CAD build for the part. Positions are in the model's coordinates, mm. Face numbers are marked on the shaded views. A direction names the side the tool comes from. Coordinates: 2 decimals unless noted, no trailing zeros. Loops run counter-clockwise (first coordinate to the right, second up) from the corner with the lowest first, then second, coordinate; pieces in that order, holes last.
1) Saw through at D-D, the plane z = -170. Give the number of separate pieces and of enclosed holes in the cut face, and give its area (3 significant figures).
2) Pin check, flat tips, straight feed: pin 1 Ø4 at (x, y) = (111.5, 10.5) entering from -Z; pin 2 Ø18 at (x, y) = (200, -78) entering from +Z; pin 3 Ø22 at (y, z) = (-3, -300) entering from +X. Stop position of each tip, or through.
3) Saw through at B-B, the plane y = -82.5. Write the cut outline in (x, z).
4) Saw through at A-A, the plane x = 208. Write the cut outline in (y, z).
5) Which spindle directions (+Z, -Z, +X, -X, +Y, -Y) get a long thin tool onto all of the face, cutting with end or side? Do the marked faces 4, 5, 6 and 7. Say none if no direction does.
6) Wall check: line 1 along Y through (x, z) = (0, -9.5); line 2 along Z through (x, y) = (193, -15.5); line 3 along Y through (x, z) = (135.5, -204.5). Give the ranges that are in metal, low to high.
7) Saw through at C-C, the plane z = -127. Write the cut outline in (x, y), and give its area (3 significant figures).
8) Two-plate mould, pull along X, no slides. Class the marked faces 1, 2 and 3: +X half, -X half, draft (parallel to the pull), parting line (faces both ways), or undercut.
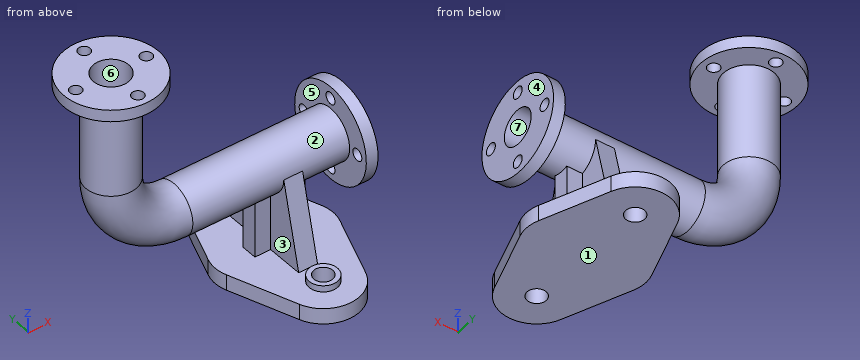
```python
from build123d import *

# Parameters (mm, degrees)
SWEEP_THIN1_PROFILE_R    = 32
SWEEP_THIN1_PROFILE_R_2  = 22.5
BOSS_EXTRUDE1_START      = -15
SKETCH14_R               = 60
SKETCH14_R_2             = 22.5
SKETCH14_R_3             = 7.5
BOSS_EXTRUDE1_DEPTH      = 15
BOSS_EXTRUDE2_START      = 15
SKETCH15_R               = 60
SKETCH15_R_2             = 7.5
SKETCH15_R_3             = 22.5
BOSS_EXTRUDE2_DEPTH      = 15
SKETCH16_R               = 12
BOSS_EXTRUDE3_DEPTH      = 20
EXTRUDE_THIN1_REACH      = 455.521
EXTRUDE_THIN1_END_RADIUS = 32
SKETCH17_W               = 64
SKETCH17_H               = 20
RIB1_START               = -12
RIB1_DEPTH               = 24
SKETCH20_R               = 18
SKETCH20_R_2             = 12
BOSS_EXTRUDE4_DEPTH      = 8


# Read off the part's stored shape, not the designer's step: Rib1
with BuildPart() as part:
    # Sweep-Thin1: sweep along a path in Sketch1
    with BuildLine(Plane(origin=(0, 0, 0), x_dir=(-1, 0, 0), z_dir=(0, 1, 0))) as sweep_thin1_path:
        Line((0, 0), (0, -135))
        ThreePointArc((0, -135), (-23.431457505, -191.568542495), (-80, -215))
        Line((-80, -215), (-280, -215))
    # Sweep-Thin1 profile (on start of the path) → Sweep-Thin1 (sweep)
    with BuildSketch(Plane(origin=(0, 0, 0), x_dir=(-1, 0, 0), z_dir=(0, 0, -1))):
        Circle(SWEEP_THIN1_PROFILE_R)
        Circle(SWEEP_THIN1_PROFILE_R_2, mode=Mode.SUBTRACT)
    sweep(path=sweep_thin1_path.line)

    # Sketch14 → Boss-Extrude1 (add)
    with BuildSketch(Plane.XY.offset(BOSS_EXTRUDE1_START)):
        Circle(SKETCH14_R)
        with Locations(Location((0, 0, 0), (0, 0, 180))):
            Circle(SKETCH14_R_2, mode=Mode.SUBTRACT)
        with Locations((0, -45)):
            Circle(SKETCH14_R_3, mode=Mode.SUBTRACT)
        with Locations((-45, 0)):
            Circle(SKETCH14_R_3, mode=Mode.SUBTRACT)
        with Locations((0, 45)):
            Circle(SKETCH14_R_3, mode=Mode.SUBTRACT)
        with Locations((45, 0)):
            Circle(SKETCH14_R_3, mode=Mode.SUBTRACT)
    extrude(amount=BOSS_EXTRUDE1_DEPTH)

    # Sketch15 → Boss-Extrude2 (add)
    with BuildSketch(Plane.YZ.offset(280).offset(BOSS_EXTRUDE2_START)):
        with Locations(Location((0, -215, 0), (0, 0, 270))):
            Circle(SKETCH15_R)
        with Locations(Location((0, -260, 0), (0, 0, 270))):
            Circle(SKETCH15_R_2, mode=Mode.SUBTRACT)
        with Locations(Location((0, -215, 0), (0, 0, 270))):
            Circle(SKETCH15_R_3, mode=Mode.SUBTRACT)
        with Locations(Location((-45, -215, 0), (0, 0, 270))):
            Circle(SKETCH15_R_2, mode=Mode.SUBTRACT)
        with Locations(Location((0, -170, 0), (0, 0, 270))):
            Circle(SKETCH15_R_2, mode=Mode.SUBTRACT)
        with Locations(Location((45, -215, 0), (0, 0, 270))):
            Circle(SKETCH15_R_2, mode=Mode.SUBTRACT)
    extrude(amount=-BOSS_EXTRUDE2_DEPTH)



with BuildPart() as body_2:
    # Sketch16 → Boss-Extrude3 (new body)
    with BuildSketch(Plane(origin=(0, 0, -340), x_dir=(0, -1, 0), z_dir=(0, 0, 1))):
        with BuildLine():
            Line((15.39090645, 280.313712262), (97.89090645, 250.286167935))
            ThreePointArc((97.89090645, 250.286167935), (127.5, 208), (97.89090645, 165.713832065))
            Line((97.89090645, 165.713832065), (15.39090645, 135.686287738))
            ThreePointArc((15.39090645, 135.686287738), (0, 132.972455673), (-15.39090645, 135.686287738))
            Line((-15.39090645, 135.686287738), (-97.89090645, 165.713832065))
            ThreePointArc((-97.89090645, 165.713832065), (-127.5, 208), (-97.89090645, 250.286167935))
            Line((-97.89090645, 250.286167935), (-15.39090645, 280.313712262))
            ThreePointArc((-15.39090645, 280.313712262), (0, 283.027544327), (15.39090645, 280.313712262))
        make_face()
        with Locations(Location((82.5, 208, 0), (0, 0, 90))):
            Circle(SKETCH16_R, mode=Mode.SUBTRACT)
        with Locations(Location((-82.5, 208, 0), (0, 0, 90))):
            Circle(SKETCH16_R, mode=Mode.SUBTRACT)
    extrude(amount=BOSS_EXTRUDE3_DEPTH)


with BuildPart() as part_1:
    add(part.part)

    add(body_2.part)  # Extrude-Thin1 merges body 2
    # Extrude-Thin1: up to this cylinder (the profile starts outside it)
    extrude_thin1_end = Plane(origin=(208, 0, -215), z_dir=(1, 0, 0)) * Cylinder(EXTRUDE_THIN1_END_RADIUS, 976.042, mode=Mode.PRIVATE)
    # Sketch17 → Extrude-Thin1 (add, up to the surface)
    with BuildSketch(Plane.XY.offset(-320), mode=Mode.PRIVATE) as extrude_thin1_sk1:
        with Locations((208, 0)):
            Rectangle(SKETCH17_W, SKETCH17_H)
    extrude_thin1_tool1 = extrude(extrude_thin1_sk1.sketch, amount=EXTRUDE_THIN1_REACH, mode=Mode.PRIVATE) - extrude_thin1_end
    add(extrude_thin1_tool1.solids().sort_by_distance((208, 0, -320))[0])

    # Rib1 outline → Rib1 (add)
    with BuildSketch(Plane.YZ.offset(208).offset(RIB1_START)):
        with BuildLine():
            Line((57, -320), (32, -215))
            ThreePointArc((32, -215), (25.922962794, -233.761663039), (10, -245.397368307))
            Line((10, -245.397368307), (10, -320))
            Line((10, -320), (57, -320))
        make_face()
    rib1 = extrude(amount=RIB1_DEPTH)

    # Mirror1: Rib1 across plane
    add(rib1.mirror(Plane.ZX))

    # Sketch20 → Boss-Extrude4 (add)
    # profile 1 of 2: a face of its own
    with BuildSketch(Plane.XY.offset(-320)):
        with Locations(Location((208, 82.5, 0), (0, 0, 180))):
            Circle(SKETCH20_R)
        with Locations((208, 82.5)):
            Circle(SKETCH20_R_2, mode=Mode.SUBTRACT)
    # profile 2 of 2: a face of its own
    with BuildSketch(Plane.XY.offset(-320)):
        with Locations(Location((208, -82.5, 0), (0, 0, 180))):
            Circle(SKETCH20_R)
        with Locations((208, -82.5)):
            Circle(SKETCH20_R_2, mode=Mode.SUBTRACT)
    extrude(amount=BOSS_EXTRUDE4_DEPTH)


solid = part_1.part
```
Data:
1. separate pieces: 3
1. enclosed holes: 1
1. area: 2,840 mm2
2. pin 1: stops at z = -245.85
2. pin 2: stops at z = -312
2. pin 3: stops at x = 240
3. outline: (160.11, -340) - (196, -340) - (196, -312) - (190, -312) - (190, -320) - (160.11, -320) - close; (220, -340) - (255.89, -340) - (255.89, -320) - (226, -320) - (226, -312) - (220, -312) - close
4. outline: (-127.5, -340) - (-94.5, -340) - (-94.5, -312) - (-100.5, -312) - (-100.5, -320) - (-127.5, -320) - close; (-70.5, -340) - (70.5, -340) - (70.5, -312) - (64.5, -312) - (64.5, -320) - (57, -320) - (32, -215) arc R32 ccw to (-32, -215) - (-57, -320) - (-64.5, -320) - (-64.5, -312) - (-70.5, -312) - close; (94.5, -340) - (127.5, -340) - (127.5, -320) - (100.5, -320) - (100.5, -312) - (94.5, -312) - close; hole circle Ø45 at (0, -215)
5. face 4: +Z, -Z, +X, +Y, -Y
5. face 5: none
5. face 6: +Z
5. face 7: +X
6. line 1: y = -60 to -52.5, -37.5 to -22.5, 22.5 to 37.5, 52.5 to 60
6. line 2: z = -340 to -320, -243 to -231.31, -198.69 to -187
6. line 3: y = -30.23 to -19.9, 19.9 to 30.23
7. outline: circle Ø64 at (0, 0); hole circle Ø45 at (0, 0)
7. area: 1,630 mm2
8. face 1: draft
8. face 2: undercut
8. face 3: -X half
